from build123d import *

# Parameters (mm, degrees)
SKETCH_1_R      = 1.5
SKETCH_1_W      = 5.4
SKETCH_1_H      = 2.8
EXTRUDE_1_DEPTH = 1.6


with BuildPart() as part:
    # 스케치1 → 보스-돌출1 (new body)
    with BuildSketch(Plane(origin=(0, 0, 0), x_dir=(1, 0, 0), z_dir=(0, 1, 0))):
        with BuildLine():
            Line((-10, 5.634530717), (10, 5.634530717))
            Line((10, 5.634530717), (10, -4.207222136))
            ThreePointArc((10, -4.207222136), (9.845653495, -4.740954435), (9.430259666, -5.109927304))
            add(Edge.make_bspline(
                [(-9.428195587, -5.109155368), (-6.286031575, -6.598013928), (-0.00904299, -8.087277746), (6.306496469, -6.598817984), (9.430259666, -5.109927304)],
                knots=[0.028590221, 0.028590221, 0.028590221, 0.028590221, 0.499914822, 0.971328473, 0.971328473, 0.971328473, 0.971328473], degree=3))
            ThreePointArc((-9.428195587, -5.109155368), (-9.845043072, -4.740167522), (-10, -4.205469283))
            Line((-10, -4.205469283), (-10, 5.634530717))
        make_face()
        with Locations(Location((0.025, -4.205469283, 0), (0, 0, 270))):
            Circle(SKETCH_1_R, mode=Mode.SUBTRACT)
        with Locations((6.175, 3.034530717)):
            Rectangle(SKETCH_1_W, SKETCH_1_H, mode=Mode.SUBTRACT)
        with Locations((-6.175, 3.034530717)):
            Rectangle(SKETCH_1_W, SKETCH_1_H, mode=Mode.SUBTRACT)
    extrude(amount=EXTRUDE_1_DEPTH)


solid = part.part
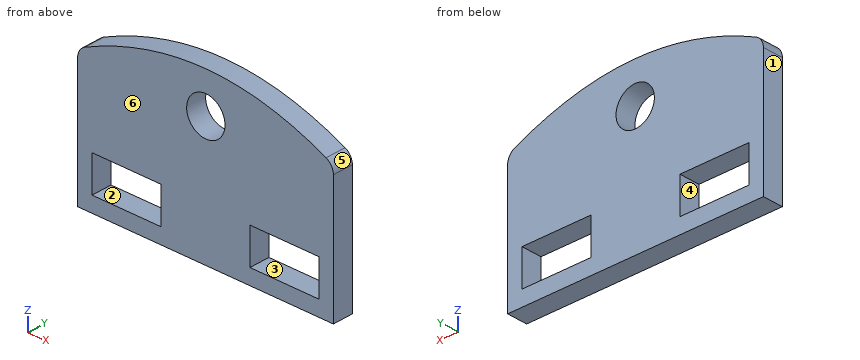
Verification items for the finished model (mm, model axes). Face numbers are marked on the shaded views. A direction names the side the tool comes from. Round coordinates to 2 decimals unless told otherwise and drop trailing zeros. Order: outer loops, then holes, each group sorted by start corner. A loop starts at its lowest first (then second) coordinate and runs counter-clockwise, first axis right, second up. Notation, with made-up numbers: (-19.5, -39.75) -> (26.5, -39.75) arc R21 cw to (26.5, -19.75) -> close; hole circle Ø6 at (65, 88). An arc over 180 degrees is marked (long way). Put each result on its own line as item: value.
1) Material ranges on line 1 (X direction, y = 0.35, z = -3.5) (3 decimals); line 2 (X direction, y = 0.5, z = 4.5); line 3 (Z direction, x = -5.25, y = 0.25), recorded low to high.
Final values:
line 1: x = -10 to -8.875, -3.475 to 3.475, 8.875 to 10
line 2: x = -9.96 to -1.45, 1.5 to 9.96
line 3: z = -5.63 to -4.43, -1.63 to 6.65
2) Mould release check, pull along X, two halves, no side actions. Record for the marked faces 3, 4, 5 and 6: +X half, -X half, draft (parallel to the pull), parting line (faces both ways), or undercut.
Final values:
face 3: undercut
face 4: undercut
face 5: +X half
face 6: draft
3) Section check C-C (y = 0.3). Give the number of separate pieces and of enclosed holes in the cut face, then the cut area to 3 significant figures.
Final values:
separate pieces: 1
enclosed holes: 3
area: 205 mm^2
4) Section check B-B (z = 3.5). Record the cut outline in (x, y).
Final values:
outline: (-10, 0) -> (-1.3, 0) -> (-1.3, 1.6) -> (-10, 1.6) -> close; (1.35, 0) -> (10, 0) -> (10, 1.6) -> (1.35, 1.6) -> close
5) Set-up check for the marked faces 1 and 2: record each of +Z, -Z, +X, -X, +Y, -Y from which the full face is reachable in a straight line by a thin tool's end or side.
Final values:
face 1: +Z, -Z, -X, +Y, -Y
face 2: +Y, -Y
6) Depth check by flat-ended pin: pin 1 (0.5 mm diameter, centred on x = -5, y = 0.5, fed in from +Z). Enter the tip coordinate at first touch or a pass-through.
Final values:
pin 1: stops at z = 6.78
7) Section check A-A (z = -3). Record the cut outline in (x, y) (3 decimals), then the cut area to 3 significant figures.
Final values:
outline: (-10, 0) -> (-8.875, 0) -> (-8.875, 1.6) -> (-10, 1.6) -> close; (-3.475, 0) -> (3.475, 0) -> (3.475, 1.6) -> (-3.475, 1.6) -> close; (8.875, 0) -> (10, 0) -> (10, 1.6) -> (8.875, 1.6) -> close
area: 14.7 mm^2
